Can you work these out from the model? Positions are in its coordinate system, mm. A direction names the side the tool comes from. Give positions to 0.01 mm unless a question says otherwise; leave off trailing zeros. Write each loop counter-clockwise with the first axis right and the second up, starting at its lowest first coordinate (ties: lowest second). Pieces come first, ordered by that corner, then holes.
from build123d import *

# Parameters (mm, degrees)
SKETCH1_R           = 1.925
BOSS_EXTRUDE1_DEPTH = 1.65
FILLET4_R           = 1
FILLET3_R           = 1.5
FILLET5_R           = 1


with BuildPart() as part:
    # Sketch1 → Boss-Extrude1 (new body)
    with BuildSketch(Plane(origin=(0, 0, 0), x_dir=(1, 0, 0), z_dir=(0, 1, 0))):
        with BuildLine():
            Line((-41.448800006, 34.091704203), (-34.091704203, 41.448800006))
            Line((-34.091704203, 41.448800006), (-0.825, 41.448800006))
            Line((-0.825, 41.448800006), (-0.825, 52.97029458))
            ThreePointArc((-0.825, 52.97029458), (0, 60.023800006), (0.825, 52.97029458))
            Line((0.825, 52.97029458), (0.825, 41.448800006))
            Line((0.825, 41.448800006), (34.091704203, 41.448800006))
            Line((34.091704203, 41.448800006), (41.448800006, 34.091704203))
            Line((41.448800006, 34.091704203), (41.448800006, 0.825))
            Line((41.448800006, 0.825), (67.97029458, 0.825))
            ThreePointArc((67.97029458, 0.825), (75.023800006, 0), (67.97029458, -0.825))
            Line((67.97029458, -0.825), (41.448800006, -0.825))
            Line((41.448800006, -0.825), (41.448800006, -34.091704203))
            Line((41.448800006, -34.091704203), (34.091704203, -41.448800006))
            Line((34.091704203, -41.448800006), (0.825, -41.448800006))
            Line((0.825, -41.448800006), (0.825, -57.97029458))
            ThreePointArc((0.825, -57.97029458), (0, -65.023800006), (-0.825, -57.97029458))
            Line((-0.825, -57.97029458), (-0.825, -41.448800006))
            Line((-0.825, -41.448800006), (-34.091704203, -41.448800006))
            Line((-34.091704203, -41.448800006), (-41.448800006, -34.091704203))
            Line((-41.448800006, -34.091704203), (-41.448800006, -0.825))
            Line((-41.448800006, -0.825), (-67.97029458, -0.825))
            ThreePointArc((-67.97029458, -0.825), (-75.023800006, 0), (-67.97029458, 0.825))
            Line((-67.97029458, 0.825), (-41.448800006, 0.825))
            Line((-41.448800006, 0.825), (-41.448800006, 34.091704203))
        make_face()
        with Locations((0, 56.448800006)):
            Circle(SKETCH1_R, mode=Mode.SUBTRACT)
        with Locations((71.448800006, 0)):
            Circle(SKETCH1_R, mode=Mode.SUBTRACT)
        with Locations((0, -61.448800006)):
            Circle(SKETCH1_R, mode=Mode.SUBTRACT)
        with Locations((-71.448800006, 0)):
            Circle(SKETCH1_R, mode=Mode.SUBTRACT)
        Polygon((-39.798800006, 33.408251825), (-33.408251825, 39.798800006), (-29.292890359, 39.798800006), (-39.798800006, 29.292890359), align=None, mode=Mode.SUBTRACT)
        Polygon((-33.408251825, -39.798800006), (-29.292890359, -39.798800006), (-39.798800006, -29.292890359), (-39.798800006, -33.408251825), align=None, mode=Mode.SUBTRACT)
        Polygon((39.798800006, -33.408251825), (39.798800006, -29.292890359), (29.292890359, -39.798800006), (33.408251825, -39.798800006), align=None, mode=Mode.SUBTRACT)
        Polygon((33.408251825, 39.798800006), (39.798800006, 33.408251825), (39.798800006, 29.292890359), (29.292890359, 39.798800006), align=None, mode=Mode.SUBTRACT)
        Polygon((-39.798800006, 26.959437981), (-26.959437981, 39.798800006), (26.959437981, 39.798800006), (39.798800006, 26.959437981), (39.798800006, -26.959437981), (26.959437981, -39.798800006), (-26.959437981, -39.798800006), (-39.798800006, -26.959437981), align=None, mode=Mode.SUBTRACT)
    extrude(amount=BOSS_EXTRUDE1_DEPTH)

    # Fillet4
    fillet4_edges = [part.edges().sort_by_distance(p)[0] for p in [
        (-0.825, 0.825, -41.448800006),
        (-0.825, 0.825, -52.97029458),
        (0.825, 0.825, -52.97029458),
        (0.825, 0.825, -41.448800006),
        (41.448800006, 0.825, -0.825),
        (67.97029458, 0.825, -0.825),
        (67.97029458, 0.825, 0.825),
        (41.448800006, 0.825, 0.825),
        (0.825, 0.825, 41.448800006),
        (0.825, 0.825, 57.97029458),
        (-0.825, 0.825, 57.97029458),
        (-0.825, 0.825, 41.448800006),
        (-41.448800006, 0.825, 0.825),
        (-67.97029458, 0.825, 0.825),
        (-67.97029458, 0.825, -0.825),
        (-41.448800006, 0.825, -0.825),
    ]]
    fillet(fillet4_edges, radius=FILLET4_R)

    # Fillet3
    fillet3_edges = [part.edges().sort_by_distance(p)[0] for p in [
        (-29.292890359, 0.825, 39.798800006),
        (-39.798800006, 0.825, 29.292890359),
        (-39.798800006, 0.825, -29.292890359),
        (-29.292890359, 0.825, -39.798800006),
        (29.292890359, 0.825, -39.798800006),
        (39.798800006, 0.825, -29.292890359),
        (39.798800006, 0.825, 29.292890359),
        (29.292890359, 0.825, 39.798800006),
    ]]
    fillet(fillet3_edges, radius=FILLET3_R)

    # Fillet5
    fillet5_edges = [part.edges().sort_by_distance(p)[0] for p in [
        (-39.798800006, 0.825, -26.959437981),
        (-39.798800006, 0.825, 26.959437981),
        (-26.959437981, 0.825, 39.798800006),
        (26.959437981, 0.825, 39.798800006),
        (39.798800006, 0.825, 26.959437981),
        (39.798800006, 0.825, -26.959437981),
        (26.959437981, 0.825, -39.798800006),
        (-26.959437981, 0.825, -39.798800006),
        (-41.448800006, 0.825, -34.091704203),
        (-34.091704203, 0.825, -41.448800006),
        (34.091704203, 0.825, -41.448800006),
        (41.448800006, 0.825, -34.091704203),
        (41.448800006, 0.825, 34.091704203),
        (34.091704203, 0.825, 41.448800006),
        (-34.091704203, 0.825, 41.448800006),
        (-41.448800006, 0.825, 34.091704203),
    ]]
    fillet(fillet5_edges, radius=FILLET5_R)


solid = part.part
(1) If I drill on L1, parallel to Z at x = 0, y = 0.7; L2, parallel to X at y = 0.4, z = 11, over which ranges is the centre line in solid material (lowest first)?
Returned:
L1: z = -60.02 to -58.37, -54.52 to -39.8, 39.8 to 59.52, 63.37 to 65.02
L2: x = -41.45 to -39.8, 39.8 to 41.45
(2) If we mould it in two halves opening along Z, with no side actions, what happens to faces 3 (the face through (36.559, 0.813, 36.648)), 4 (the face through (-0.42, 0.81, -54.57)), 5 (the face through (-37.72, 0.81, 37.82)), 6 (the face through (-75.02, 0.81, 0.14))? For each: +Z half, -Z half, draft (parallel to the pull), parting line (faces both ways), or undercut.
Returned:
face 3: undercut
face 4: undercut
face 5: +Z half
face 6: parting line
(3) For faces 1 (the face through (0, 0, -44)), 2 (the face through (34.58, 0.81, 34.51)), which set-ups out of +Z, -Z, +X, -X, +Y, -Y let a thin tool reach every point of the face, with its end or its side?
Returned:
face 1: +Z, -Z, +X, -X, -Y
face 2: +Y, -Y
(4) Will these pins go through, and if not, where does the flat tip stop? P1, Ø3, axis at x = 0, z = 61.45, coming from the +Y side; P2, Ø0.8, axis at x = 14, y = 0.5, coming from the +Z side; P3, Ø0.5, axis at x = -53, y = 0.5, coming from the +Z side (3 decimals); P4, Ø5, axis at x = 71.45, z = 0, coming from the -Y side.
Returned:
P1: passes through
P2: stops at z = 41.45
P3: stops at z = 0.825
P4: stops at y = 0
(5) Imagine slicing it at B-B, the plane x = 17. Write out the boundary of the cut face in (y, z), plus the area to 4 significant figures.
Returned:
outline: (0, -41.45) - (1.65, -41.45) - (1.65, -39.8) - (0, -39.8) - close; (0, 39.8) - (1.65, 39.8) - (1.65, 41.45) - (0, 41.45) - close
area: 5.445 mm2
(6) Imagine slicing it at A-A, the plane z = 9.5. Write out the boundary of the cut face in (x, y), plus the area to 4 significant figures.
Returned:
outline: (-41.45, 0) - (-39.8, 0) - (-39.8, 1.65) - (-41.45, 1.65) - close; (39.8, 0) - (41.45, 0) - (41.45, 1.65) - (39.8, 1.65) - close
area: 5.445 mm2
(7) Imagine slicing it at D-D, the plane y = 0.9. Give the number of separate pieces and of enclosed holes in the cut face, plus the area to 3 significant figures.
Returned:
separate pieces: 1
enclosed holes: 9
area: 891 mm2
(8) Imagine slicing it at C-C, the plane z = -49.5. Write out the boundary of the cut face in (x, y) (3 decimals).
Returned:
outline: (-0.825, 0) - (0.825, 0) - (0.825, 1.65) - (-0.825, 1.65) - close
